Part model, mm, in its own coordinate system. A direction names the side the tool comes from. Round coordinates to 2 decimals unless told otherwise and drop trailing zeros. Loops run counter-clockwise (first coordinate to the right, second up) from the corner with the lowest first, then second, coordinate; pieces in that order, holes last. Notation, with made-up numbers: (4, 74.25) -> (50, 74.25) arc R11 cw to (50, 83.25) -> close; hole circle Ø11 at (-25, 1.25). An arc over 180 degrees is marked (long way). Use a Markdown table: item, result. Add a question column.
Item 1: Cut at C-C, the plane z = 152.5. List the corners of the cut face in (x, y) (3 decimals).
Item 2: Probe line 1 (Y direction, x = 14, z = 108.5) (3 decimals); line 2 (X direction, y = -26, z = 155.5) (3 decimals); line 3 (X direction, y = -47, z = 134). List the from-to ranges inside material, lowest first. Write a range as [from, to].
Item 3: Two-plate mould, pull along Y, no slides. Class faces 3 (the face through (4.703, -4.624, 128.778)), 4 (the face through (50.8, -26, 125)), 5 (the face through (25, -50.8, 125)): pulls with the +Y half, pulls with the -Y half, needs draft (parallel to the pull), parting line crosses it, or undercut.
Item 4: Cut at B-B, the plane y = -20.5. List the corners of the cut face in (x, z) (3 decimals).
Item 5: Which spindle directions (+Z, -Z, +X, -X, +Y, -Y) get a long thin tool onto all of the face, cutting with end or side? Do faces 1 (the face through (46.176, -4.703, 128.778)), 2 (the face through (49.272, -1.449, 128.778)). Say none if no direction does.
Item 6: Cut at A-A, the plane x = 35. List the corners of the cut face in (y, z) (3 decimals), plus the area to 3 significant figures.
```python
from build123d import *

# Parameters (mm, degrees)
F0_W     = 50.8
F0_H     = 50.8
F0_W_2   = 44.45
F0_H_2   = 44.45
F1_DEPTH = 254
F2_R     = 5.08


with BuildPart() as f1:
    # F0 (on Top) → F1 (new body)
    with BuildSketch(Plane.XY):
        with Locations((25.4, -25.4)):
            Rectangle(F0_W, F0_H)
        with Locations((25.4, -25.4)):
            Rectangle(F0_W_2, F0_H_2, mode=Mode.SUBTRACT)
    extrude(amount=F1_DEPTH)

    # F2
    f2_edges = [f1.edges().sort_by_distance(p)[0] for p in [
        (50.8, -50.8, 127),
        (0, -50.8, 127),
        (50.8, 0, 127),
        (0, 0, 127),
        (47.625, -3.175, 127),
        (3.175, -3.175, 127),
        (3.175, -47.625, 127),
        (47.625, -47.625, 127),
    ]]
    fillet(f2_edges, radius=F2_R)


solid = f1.part
```
A:
| question | item | result |
|---|---|---|
| 1 | outline | (0, -45.72) arc R5.08 ccw to (5.08, -50.8) -> (45.72, -50.8) arc R5.08 ccw to (50.8, -45.72) -> (50.8, -5.08) arc R5.08 ccw to (45.72, 0) -> (5.08, 0) arc R5.08 ccw to (0, -5.08) -> close; hole (3.175, -42.545) arc R5.08 ccw to (8.255, -47.625) -> (42.545, -47.625) arc R5.08 ccw to (47.625, -42.545) -> (47.625, -8.255) arc R5.08 ccw to (42.545, -3.175) -> (8.255, -3.175) arc R5.08 ccw to (3.175, -8.255) -> close |
| 2 | line 1 | y = [-50.8, -47.625], [-3.175, 0] |
| 2 | line 2 | x = [0, 3.175], [47.625, 50.8] |
| 2 | line 3 | x = [0.16, 5.81], [44.99, 50.64] |
| 3 | face 3 | undercut |
| 3 | face 4 | needs draft |
| 3 | face 5 | pulls with the -Y half |
| 4 | outline | (0, 0) -> (3.175, 0) -> (3.175, 254) -> (0, 254) -> close; (47.625, 0) -> (50.8, 0) -> (50.8, 254) -> (47.625, 254) -> close |
| 5 | face 1 | +Z, -Z |
| 5 | face 2 | +Z, -Z, +X, +Y |
| 6 | outline | (-50.8, 0) -> (-47.625, 0) -> (-47.625, 254) -> (-50.8, 254) -> close; (-3.175, 0) -> (0, 0) -> (0, 254) -> (-3.175, 254) -> close |
| 6 | area | 1,610 mm^2 |
